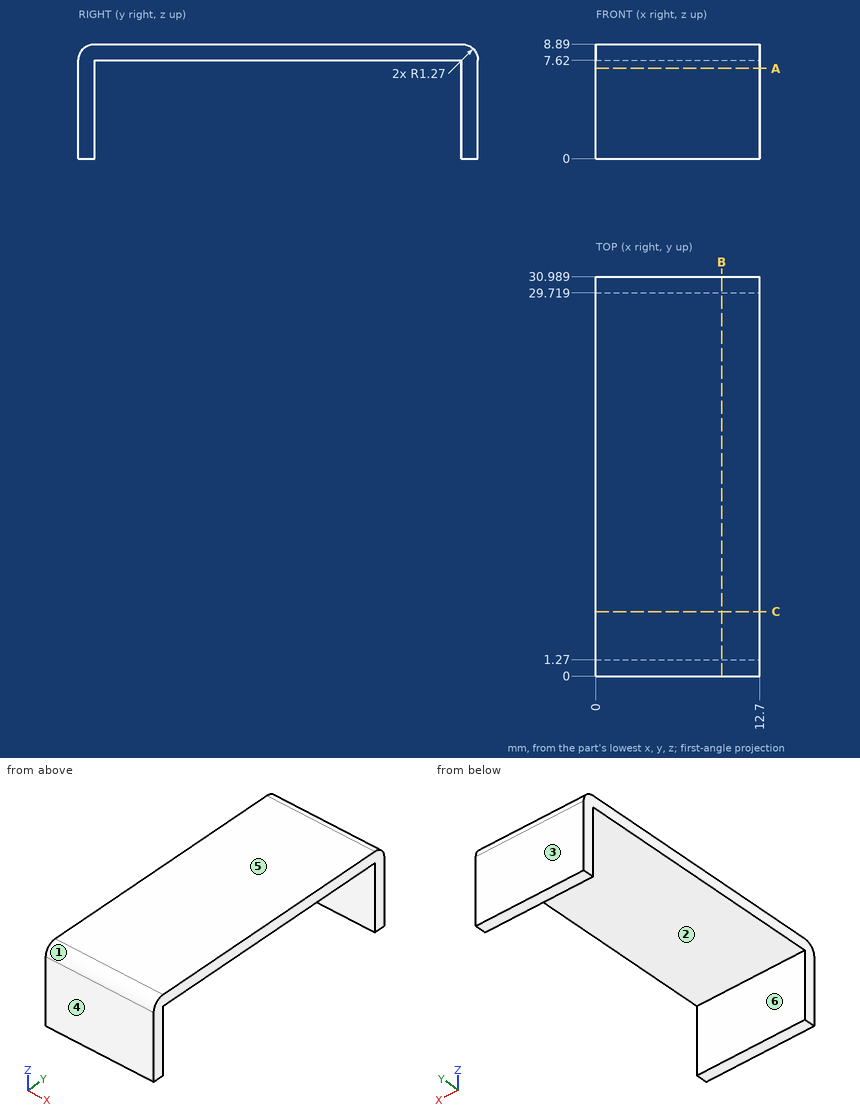
Geometry: see drawing. Coordinates: mm, zero at the bounding-box minimum. A direction names the side the tool comes from. Coordinates: 2 decimals unless noted, no trailing zeros. Loops run counter-clockwise (first coordinate to the right, second up) from the corner with the lowest first, then second, coordinate; pieces in that order, holes last. Notation, with made-up numbers: (80, 1.25) - (84, 1.25) arc R29 cw to (84, 24.25) - close; hole circle Ø7 at (10, -18.75). An arc over 180 degrees is marked (long way). Return JSON: item names as keys, results as strings.
Q1. Mould query, pull axis Y, two halves, no side actions, for the marked faces 3, 4, 5 and 6. Classes: released by +Y, released by -Y, zero draft, split by the parting line, or undercut.
Results:
{"face 3": "released by +Y", "face 4": "released by -Y", "face 5": "zero draft", "face 6": "undercut"}
Q2. Section B-B, the plane x = 9.75. Return loops of the section in (y, z).
Results:
{"outline": "(0, 0) - (1.27, 0) - (1.27, 7.62) - (29.72, 7.62) - (29.72, 0) - (30.99, 0) - (30.99, 7.62) arc R1.27 ccw to (29.72, 8.89) - (1.27, 8.89) arc R1.27 ccw to (0, 7.62) - close"}
Q3. Contact query for a flat-ended pin moving along its axis: P1, Ø4, axis at x = 9, y = 14, coming from the -Z side. Output: stop coordinate, or through.
Results:
{"P1": "z = 7.62"}
Q4. Section A-A, the plane z = 7. Return loops of the section in (x, y).
Results:
{"outline": "(0, 0) - (12.7, 0) - (12.7, 1.27) - (0, 1.27) - close; (0, 29.72) - (12.7, 29.72) - (12.7, 30.99) - (0, 30.99) - close"}
Q5. Access query for the marked faces 1 and 2. Directions: +Z, -Z, +X, -X, +Y, -Y. A direction counts if a zero-diameter tool reaches every point of the face in a straight line with its end or side. Return the directions, or none.
Results:
{"face 1": "+Z, +X, -X, -Y", "face 2": "-Z, +X, -X"}
Q6. Material intervals for line 1 along Y through (x, z) = (0.5, 6.75); line 2 along Z through (x, y) = (10.5, 2); line 3 along Y through (x, z) = (10, 7.75), sorted ascending.
Results:
{"line 1": "0 to 1.27, 29.72 to 30.99", "line 2": "7.62 to 8.89", "line 3": "0.01 to 30.98"}
Q7. Section C-C, the plane y = 5. Return loops of the section in (x, z).
Results:
{"outline": "(0, 7.62) - (12.7, 7.62) - (12.7, 8.89) - (0, 8.89) - close"}
